Geometry check sheet. Reference: the model listing, model coordinates, mm. A direction names the side the tool comes from. Give positions to 0.01 mm unless a question says otherwise; leave off trailing zeros. Loops run counter-clockwise (first coordinate to the right, second up) from the corner with the lowest first, then second, coordinate; pieces in that order, holes last. Notation, with made-up numbers: (-1.5, 18) -> (10.5, 18) arc R21 cw to (10.5, 53) -> close; hole circle Ø1 at (49, 38). An arc over 180 degrees is marked (long way). One line per question, with ' | ' between items.
from build123d import *

# Parameters (mm, degrees)
SKETCH1_R           = 7.6
SKETCH1_R_2         = 6.6
BOSS_EXTRUDE1_DEPTH = 25
BOSS_EXTRUDE2_START = -5
SKETCH2_R           = 1.625
SKETCH2_R_2         = 1.5
BOSS_EXTRUDE2_DEPTH = 5
FILLET1_R           = 10
FILLET2_R           = 2.5


with BuildPart() as part:
    # Sketch1 → Boss-Extrude1 (new body)
    with BuildSketch(Plane(origin=(0, 0, 0), x_dir=(1, 0, 0), z_dir=(0, 1, 0))):
        with Locations(Location((0, 0, 0), (0, 0, 270))):
            Circle(SKETCH1_R)
        with Locations(Location((0, 0, 0), (0, 0, 270))):
            Circle(SKETCH1_R_2, mode=Mode.SUBTRACT)
    extrude(amount=BOSS_EXTRUDE1_DEPTH)

    # Sketch2 → Boss-Extrude2 (add)
    # profile 1 of 2: a face of its own
    with BuildSketch(Plane(origin=(0, 25, 0), x_dir=(1, 0, 0), z_dir=(0, 1, 0)).offset(BOSS_EXTRUDE2_START)):
        with BuildLine():
            Line((-6.108191222, 2.5), (-15, 2.5))
            Line((-15, 2.5), (-15, -2.5))
            Line((-15, -2.5), (-6.108191222, -2.5))
            ThreePointArc((-6.108191222, -2.5), (-6.6, 0), (-6.108191222, 2.5))
        make_face()
        with Locations(Location((-12.5, 0, 0), (0, 0, 270))):
            Circle(SKETCH2_R, mode=Mode.SUBTRACT)
    # profile 2 of 2: a face of its own
    with BuildSketch(Plane(origin=(0, 25, 0), x_dir=(1, 0, 0), z_dir=(0, 1, 0)).offset(BOSS_EXTRUDE2_START)):
        with BuildLine():
            Line((15, -2.5), (6.108191222, -2.5))
            ThreePointArc((6.108191222, -2.5), (6.6, 0), (6.108191222, 2.5))
            Line((6.108191222, 2.5), (15, 2.5))
            Line((15, 2.5), (15, -2.5))
        make_face()
        with Locations(Location((12.5, 0, 0), (0, 0, 270))):
            Circle(SKETCH2_R_2, mode=Mode.SUBTRACT)
    extrude(amount=BOSS_EXTRUDE2_DEPTH)

    # Fillet1
    fillet1_edges = [part.edges().sort_by_distance(p)[0] for p in [
        (-7.177046746, 22.5, -2.5),
        (-7.177046746, 22.5, 2.5),
        (7.177046746, 22.5, 2.5),
        (7.177046746, 22.5, -2.5),
    ]]
    fillet(fillet1_edges, radius=FILLET1_R)

    # Fillet2
    fillet2_edges = [part.edges().sort_by_distance(p)[0] for p in [
        (15, 22.5, 2.5),
        (15, 22.5, -2.5),
        (-15, 22.5, 2.5),
        (-15, 22.5, -2.5),
    ]]
    fillet(fillet2_edges, radius=FILLET2_R - 0.0001)  # a hair under: the kernel refuses the full size


solid = part.part
Item 1: Sectioned sample at C-C (y = 22.5). Give the number of separate pieces and of enclosed holes in the cut face, plus the area to 3 significant figures.
Result:
separate pieces: 1 | enclosed holes: 3 | area: 112 mm2
Item 2: Scan lines: probe 1 along Z at (x, y) = (0, 9.75); probe 2 along Z at (x, y) = (3, 13.5). Record each from-to range of solid material in increasing order.
Result:
probe 1: -7.6 to -6.6, 6.6 to 7.6 | probe 2: -6.98 to -5.88, 5.88 to 6.98
Item 3: Set-up check for faces 1 (the face through (0.334, 12.325, -7.593)), 2 (the face through (7, 25, -1)): record each of +Z, -Z, +X, -X, +Y, -Y from which the full face is reachable in a straight line by a thin tool's end or side.
Result:
face 1: -Y | face 2: +Z, -Z, +X, -X, +Y
Item 4: Sectioned sample at D-D (y = 4.5). Record the cut outline in (x, z).
Result:
outline: circle Ø15.2 at (0, 0); hole circle Ø13.2 at (0, 0)
Item 5: Sectioned sample at B-B (z = -2). Record the cut outline in (x, y), plus the area to 3 significant figures.
Result:
outline: (-14, 20) -> (-7.33, 20) -> (-7.33, 0) -> (-6.29, 0) -> (-6.29, 25) -> (-14, 25) -> close; (6.29, 0) -> (7.33, 0) -> (7.33, 20) -> (14, 20) -> (14, 25) -> (6.29, 25) -> close | area: 119 mm2
Item 6: Sectioned sample at A-A (x = 0). Record the cut outline in (y, z), plus the area to 3 significant figures.
Result:
outline: (0, -7.6) -> (25, -7.6) -> (25, -6.6) -> (0, -6.6) -> close; (0, 6.6) -> (25, 6.6) -> (25, 7.6) -> (0, 7.6) -> close | area: 50.0 mm2
Item 7: Release check for a two-part mould opening along X. For faces 3 (the face through (-14.086, 22.465, -0.352)), 4 (the face through (-8.634, 22.465, 3.232)), 5 (the face through (14, 23, -2)), 6 (the face through (12.95, 22.46, 1.43)) record: pulls with the +X half, pulls with the -X half, needs draft (parallel to the pull), parting line crosses it, or undercut.
Result:
face 3: undercut | face 4: pulls with the -X half | face 5: pulls with the +X half | face 6: undercut
Item 8: Depth check by flat-ended pin: pin 1 Ø7.5 at (x, z) = (12, 2.5) entering from -Y; pin 2 Ø5 at (y, z) = (3, -3.5) entering from +X; pin 3 Ø4 at (y, z) = (17.5, -1) entering from -X. Enter the tip coordinate at first touch or a pass-through.
Result:
pin 1: y = 20 | pin 2: x = 7.53 | pin 3: x = -7.6
